Geometry: final body of the model. Coordinates: model frame, mm. A direction names the side the tool comes from. Coordinates: 2 decimals unless noted, no trailing zeros. Order: outer loops, then holes, each group sorted by start corner. A loop starts at its lowest first (then second) coordinate and runs counter-clockwise, first axis right, second up. Notation, with made-up numbers: M 34,14 L 68,14 A24 cw 68,40 Z; hole C 30.25,34 d8. An arc over 180 degrees is marked long. Use CSV: the item, a comma, the result in double quotes. Start each with the question number.
1. Pull-direction query (X, two-part tool) for faces 1 (the cylindrical face through (-0.401, 15.487, 1.806)), 2 (the flat face through (0, 3, 1.8)), 3 (the cylindrical face through (-0.28, 9.86, -2.13)), 4 (the conical face through (0, 4, 0)); classes: pulls with the +X half, pulls with the -X half, needs draft (parallel to the pull), parting line crosses it, or undercut.
2. Section query A-A on y = 15.75. Return the cut outline in (x, z).
3. Set-up query: faces 5 (the cylindrical face through (0.03, 1.52, -1.55)), 6 (the conical face through (0, 10, 0)). Return all of +Z, -Z, +X, -X, +Y, -Y with unobstructed straight access to the full face (end or side cutting, diameter ignored); none if empty.
4. First-contact query: P1, Ø1.5, axis at y = 16.5, z = 1, coming from the -X side; P2, Ø1.5, axis at y = 4.5, z = -1.5, coming from the -X side; P3, Ø2, axis at x = 0, z = 0.5, coming from the +Y side. Flat tips, straight axial feed; report the tip coordinate or a pass-through.
5. Material intervals for line 1 (X direction, y = 13.25, z = 0); line 2 (Z direction, x = -0.65, y = 15), sorted ascending.
6. Section query B-B on y = 6. Return the cut outline in (x, z), and give its area (3 significant figures).
from build123d import *

# Parameters (mm, degrees)
ESBO_O3_W             = 4.788650246
ESBO_O3_H             = 2.452019704
CORTE_EXTRUS_O4_DEPTH = 3
CHANFRO1_SIZE         = 0.15


with BuildPart() as part:
    # Esboço1 → Revolução1 (revolve)
    with BuildSketch(Plane.XY):
        Polygon((0, 4), (0, 10), (1.85, 11), (1.85, 20), (2.15, 20), (2.15, 0), (1.55, 0), (1.55, 3), align=None)
    revolve(axis=Axis((0, 4, 0), (0, 1, 0)))

    # Esboço3 → Corte-extrusão4 (cut)
    with BuildSketch(Plane.XZ):
        with Locations((0, 1.226009852)):
            Rectangle(ESBO_O3_W, ESBO_O3_H)
    extrude(amount=-CORTE_EXTRUS_O4_DEPTH, mode=Mode.SUBTRACT)

    # Chanfro1
    chanfro1_edges = [part.edges().sort_by_distance(p)[0] for p in [
        (-1.85, 20, 0),
    ]]
    chamfer(chanfro1_edges, length=CHANFRO1_SIZE)


solid = part.part
Results list:
1,face 1,"undercut"
1,face 2,"needs draft"
1,face 3,"parting line crosses it"
1,face 4,"undercut"
2,outline,"C 0,0 d4.3; hole C 0,0 d3.7"
3,face 5,"+Z, -Y"
3,face 6,"+Y"
4,P1,"stops at x = -2.14"
4,P2,"stops at x = -2.01"
4,P3,"stops at y = 10.81"
5,line 1,"x = -2.15 to -1.85, 1.85 to 2.15"
5,line 2,"z = -2.05 to -1.73, 1.73 to 2.05"
6,outline,"C 0,0 d4.3"
6,area,"14.5 mm²"
